Work out the finished part from the listing and answer in its coordinate system (mm). Face numbers are marked on the shaded views. A direction names the side the tool comes from. Round coordinates to 2 decimals unless told otherwise and drop trailing zeros. Loops run counter-clockwise (first coordinate to the right, second up) from the corner with the lowest first, then second, coordinate; pieces in that order, holes last. Notation, with made-up numbers: (6.5, 4.5) - (51.5, 4.5) arc R28 ccw to (51.5, 28.5) - close; hole circle Ø2 at (20.5, 0.25). An arc over 180 degrees is marked (long way). Answer as CSV lines item,"result". Start each with the question number.
Autodesk Inventor part; units mm, degrees
ref_plane "YZ Plane" through (0, 0, 0) normal (1, 0, 0) x (0, 1, 0)
ref_plane "XZ Plane" through (0, 0, 0) normal (0, 1, 0) x (-1, 0, 0)
ref_plane "XY Plane" through (0, 0, 0) normal (0, 0, 1) x (1, 0, 0)
sketch "スケッチ1" plane through (0, 0, 0) normal (0, 0, 1) x (1, 0, 0)
  line L0 (-1.75, -4.25) -> (1.75, -4.25)
  line L1 (1.75, -4.25) -> (1.75, 4.25)
  line L2 (1.75, 4.25) -> (-1.75, 4.25)
  line L3 (-1.75, 4.25) -> (-1.75, -4.25)
  line L4 (-1.75, -4.25) -> (1.75, 4.25) construction
  line L5 (1.75, -4.25) -> (-1.75, 4.25) construction
  point P0 (0, 0)
  dimension "d0" = 8.5
  dimension "d1" = 3.5
extrude "押し出し1" add sketch "スケッチ1" along normal blind 3.6
sketch "スケッチ2" plane through (0, 0, 3.6) normal (0, 0, 1) x (1, 0, 0)
  line L0 (-0.75, 1.85) -> (0.75, 1.85) construction
  line L1 (0.75, 1.85) -> (0.75, -1.85) construction
  line L2 (0.75, -1.85) -> (-0.75, -1.85) construction
  line L3 (-0.75, -1.85) -> (-0.75, 1.85) construction
  line L4 (-0.75, 1.85) -> (0.75, -1.85) construction
  line L5 (0.75, 1.85) -> (-0.75, -1.85) construction
  line L6 (-0.75, -1.85) -> (0.75, -1.85)
  line L7 (0.75, -1.85) -> (0.75, -0.35)
  line L8 (0.75, -0.35) -> (-0.75, -0.35)
  line L9 (-0.75, -0.35) -> (-0.75, -1.85)
  point P0 (0, 0)
  dimension "d4" = 3.7
  dimension "d5" = 1.5
  dimension "d6" = 1.5
extrude "押し出し2" add sketch "スケッチ2" along normal blind 5
sketch "スケッチ3" plane through (0, 0, 0) normal (0, 0, -1) x (-1, 0, 0)
  line L0 (-0.15, -2.75) -> (0.15, -2.75) construction
  line L1 (0.15, -2.75) -> (0.15, 2.75) construction
  line L2 (0.15, 2.75) -> (-0.15, 2.75) construction
  line L3 (-0.15, 2.75) -> (-0.15, -2.75) construction
  line L4 (-0.15, -2.75) -> (0.15, 2.75) construction
  line L5 (0.15, -2.75) -> (-0.15, 2.75) construction
  line L6 (-0.15, 2.75) -> (0.15, 2.75)
  line L7 (0.15, 2.75) -> (0.15, 2.25)
  line L8 (0.15, 2.25) -> (-0.15, 2.25)
  line L9 (-0.15, 2.25) -> (-0.15, 2.75)
  line L10 (-0.15, -0.25) -> (0.15, -0.25)
  line L11 (0.15, -0.25) -> (0.15, 0.25)
  line L12 (0.15, 0.25) -> (-0.15, 0.25)
  line L13 (-0.15, 0.25) -> (-0.15, -0.25)
  line L14 (-0.15, -0.25) -> (0.15, 0.25) construction
  line L15 (0.15, -0.25) -> (-0.15, 0.25) construction
  line L16 (-0.15, -2.75) -> (0.15, -2.75)
  line L17 (0.15, -2.75) -> (0.15, -2.25)
  line L18 (0.15, -2.25) -> (-0.15, -2.25)
  line L19 (-0.15, -2.25) -> (-0.15, -2.75)
  point P0 (0, 0)
  dimension "d9" = 0.3
  dimension "d10" = 5.5
  dimension "d11" = 0.5
  dimension "d12" = 0.5
  dimension "d13" = 0.5
extrude "押し出し3" add sketch "スケッチ3" along normal blind 3.6
properties part number "SS-12D00-G5"
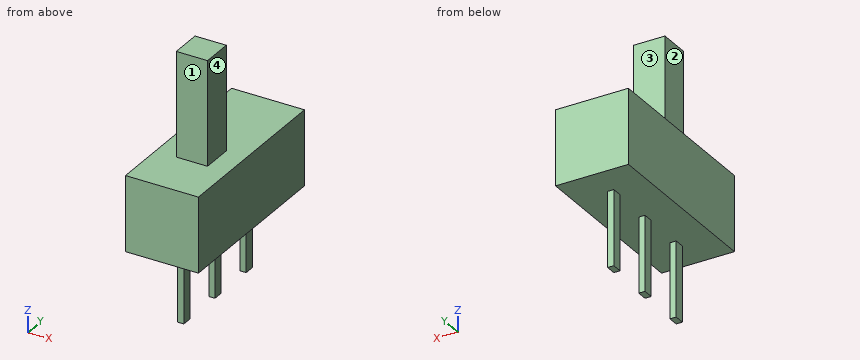
Item 1: Which of the six approach directions +Z, -Z, +X, -X, +Y, -Y give full straight-line access (tool end or side, diameter ignored) to the marked faces 1, 2, 3 and 4?
Item 2: Section C-C, the plane x = 0.45 is taken. Give the vertices of the cut face in (y, z), and give its area (3 significant figures).
Item 3: Section D-D, the plane z = 6 is taken. Give the vertices of the cut face in (x, y).
Item 4: Section B-B, the plane y = -0.75 is taken. Give the vertices of the cut face in (x, z).
Item 5: Find the intervals of material crossed by L1, parallel to Y at x = -0.2, z = 6; L2, parallel to X at y = -0.75, z = 7.25; L3, parallel to Z at x = -1.15, y = 1.5, in increasing order.
Item 6: Flat-ended cylindrical pins translate along their axes: pin 1 Ø1 at (y, z) = (3.5, 4.5) entering from -X; pin 2 Ø3 at (y, z) = (2.5, 5) entering from -X; pin 3 Ø1.2 at (y, z) = (-1.5, 7) entering from -X; pin 4 Ø1.2 at (x, z) = (0, 6) entering from -Y. Find the tip coordinate at first contact, or state that the pin passes through.
Item 7: Section A-A, the plane z = -2.75 is taken. Give the vertices of the cut face in (x, y).
Answer:
1,face 1,"+Z, +X, -X, -Y"
1,face 2,"+Z, -X, +Y, -Y"
1,face 3,"+Z, +X, -X, +Y"
1,face 4,"+Z, +X, +Y, -Y"
2,outline,"(-4.25, 0) - (4.25, 0) - (4.25, 3.6) - (-0.35, 3.6) - (-0.35, 8.6) - (-1.85, 8.6) - (-1.85, 3.6) - (-4.25, 3.6) - close"
2,area,"38.1 mm²"
3,outline,"(-0.75, -1.85) - (0.75, -1.85) - (0.75, -0.35) - (-0.75, -0.35) - close"
4,outline,"(-1.75, 0) - (1.75, 0) - (1.75, 3.6) - (0.75, 3.6) - (0.75, 8.6) - (-0.75, 8.6) - (-0.75, 3.6) - (-1.75, 3.6) - close"
5,L1,"y = -1.85 to -0.35"
5,L2,"x = -0.75 to 0.75"
5,L3,"z = 0 to 3.6"
6,pin 1,"passes through"
6,pin 2,"stops at x = -1.75"
6,pin 3,"stops at x = -0.75"
6,pin 4,"stops at y = -1.85"
7,outline,"(-0.15, -2.75) - (0.15, -2.75) - (0.15, -2.25) - (-0.15, -2.25) - close; (-0.15, -0.25) - (0.15, -0.25) - (0.15, 0.25) - (-0.15, 0.25) - close; (-0.15, 2.25) - (0.15, 2.25) - (0.15, 2.75) - (-0.15, 2.75) - close"
